Verification items for the finished model (mm, model axes). Round coordinates to 2 decimals unless told otherwise and drop trailing zeros. Loops run counter-clockwise (first coordinate to the right, second up) from the corner with the lowest first, then second, coordinate; pieces in that order, holes last.
from build123d import *

# Parameters (mm, degrees)
F0_W     = 440
F0_H     = 210
F1_DEPTH = 80
F2_SIZE2 = 60
F2_SIZE  = 20
F3_R     = 50
F4_R     = 50
F5_R     = 20
F6_R     = 20
F7_R     = 20
F8_DEPTH = 20


with BuildPart() as f1:
    # F0 (on Top) → F1 (new body)
    with BuildSketch(Plane.XY):
        with Locations((220, 105)):
            Rectangle(F0_W, F0_H)
    extrude(amount=F1_DEPTH)

    # F2
    f2_edges = [f1.edges().sort_by_distance(p)[0] for p in [
        (440, 210, 40),
        (0, 210, 40),
        (220, 210, 0),
        (220, 210, 80),
    ]]
    f2_side = f1.faces().sort_by_distance((220, 210, 40))[0]
    chamfer(f2_edges, length=F2_SIZE, length2=F2_SIZE2, reference=f2_side)

    # F3
    f3_edges = [f1.edges().sort_by_distance(p)[0] for p in [
        (20, 210, 40),
    ]]
    fillet(f3_edges, radius=F3_R)

    # F4
    f4_edges = [f1.edges().sort_by_distance(p)[0] for p in [
        (420, 210, 40),
    ]]
    fillet(f4_edges, radius=F4_R)

    # F5
    f5_edges = [f1.edges().sort_by_distance(p)[0] for p in [
        (0, 0, 40),
    ]]
    fillet(f5_edges, radius=F5_R)

    # F6
    f6_edges = [f1.edges().sort_by_distance(p)[0] for p in [
        (440, 0, 40),
    ]]
    fillet(f6_edges, radius=F6_R)

    # F7 (on face) → F8 (join)
    with BuildSketch(Plane.XZ):
        with Locations((100, 40)):
            Circle(F7_R)
        with Locations((220, 40)):
            Circle(F7_R)
        with Locations((340, 40)):
            Circle(F7_R)
    extrude(amount=F8_DEPTH)


solid = f1.part
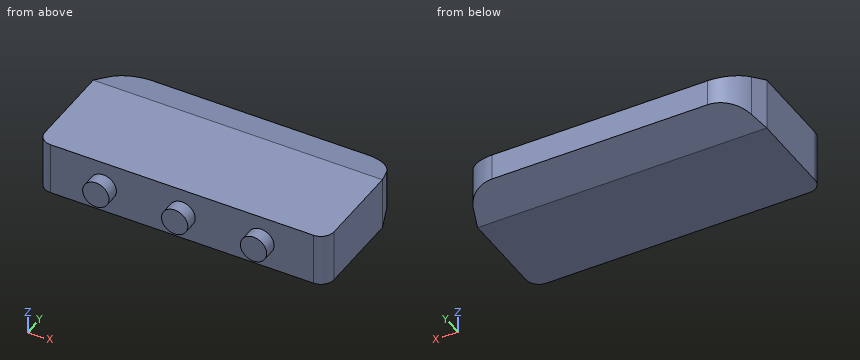
1. Section check D-D (y = 195). Enter the section's corners in (x, z), then the cut area to 3 significant figures.
2. Section check B-B (z = 40). Enter the section's corners in (x, y), then the cut area to 3 significant figures.
3. Gauge pin test, flat ends, axial feed: P1, Ø4, axis at x = 124, y = 30, coming from the -Z side; P2, Ø8, axis at y = 174.5, z = 9, coming from the -X side; P3, Ø4, axis at x = 188, z = 69, coming from the -Y side. Record the tip position at first contact, or that the pin passes through.
4. Section check A-A (x = 100). Enter the section's corners in (y, z).
5. Section check C-C (x = 297). Enter the section's corners in (y, z).
6. Scan lines: L1, parallel to Y at x = 157, z = 52.5; L2, parallel to Z at x = 149, y = 164.5; L3, parallel to Y at x = 409, z = 54. Record each from-to range of solid material in increasing order.
Taken from the geometry:
1. outline: (20.33, 15) - (419.67, 15) - (419.67, 65) - (20.33, 65) - close
1. area: 20,000 mm2
2. outline: (0, 20) arc R20 ccw to (20, 0) - (80, 0) - (80, -20) - (120, -20) - (120, 0) - (200, 0) - (200, -20) - (240, -20) - (240, 0) - (320, 0) - (320, -20) - (360, -20) - (360, 0) - (420, 0) arc R20 ccw to (440, 20) - (440, 150) - (431.4, 175.81) arc R50 ccw to (383.96, 210) - (56.04, 210) arc R50 ccw to (8.6, 175.81) - (0, 150) - close
2. area: 92,900 mm2
3. P1: stops at z = 0
3. P2: stops at x = 6.83
3. P3: stops at y = 0
4. outline: (-20, 20) - (0, 20) - (0, 0) - (150, 0) - (210, 20) - (210, 60) - (150, 80) - (0, 80) - (0, 60) - (-20, 60) - close
5. outline: (0, 0) - (150, 0) - (210, 20) - (210, 60) - (150, 80) - (0, 80) - close
6. L1: y = 0 to 210
6. L2: z = 4.83 to 75.17
6. L3: y = 0 to 203.28
